Autodesk Inventor part; units mm, degrees
ref_plane "YZ Plane" through (0, 0, 0) normal (1, 0, 0) x (0, 1, 0)
ref_plane "XZ Plane" through (0, 0, 0) normal (0, 1, 0) x (-1, 0, 0)
ref_plane "XY Plane" through (0, 0, 0) normal (0, 0, 1) x (1, 0, 0)
sketch "Náčrt1" plane through (0, 0, 0) normal (0, 0, 1) x (1, 0, 0)
  line L0 (9.3423, 0) -> (16.6577, 0)
  line L1 (26, 28.3693) -> (26, 51.0917)
  line L2 (0, 51.0917) -> (0, 28.3693)
  circle A0 centre (13, 67) radius 10
  arc A1 (23.4879, 59.3186) -> (2.5121, 59.3186) centre (13, 67) ccw
  circle A2 centre (13, 8) radius 4.5
  line L3 (10, 43) -> (16, 43)
  line L4 (16, 43) -> (16, 33)
  line L5 (16, 33) -> (10, 33)
  line L6 (10, 33) -> (10, 43)
  line L7 (26, 51.0917) -> (26, 28.3693)
  line L8 (0, 28.3693) -> (0, 51.0917)
  line L9 (0.0896, 27.6417) -> (6.4319, 2.2724)
  line L10 (25.9104, 27.6417) -> (19.5681, 2.2724)
  line L11 (25.4962, 52.7558) -> (23.4121, 55.8819)
  line L12 (0.5038, 52.7558) -> (2.5879, 55.8819)
  arc A3 (6.4319, 2.2724) -> (9.3423, 0) centre (9.3423, 3) ccw
  arc A4 (16.6577, 0) -> (19.5681, 2.2724) centre (16.6577, 3) ccw
  arc A5 (0.5038, 52.7558) -> (0, 51.0917) centre (3, 51.0917) ccw
  arc A6 (26, 51.0917) -> (25.4962, 52.7558) centre (23, 51.0917) ccw
  arc A7 (23.4879, 59.3186) -> (23.4121, 55.8819) centre (25.9082, 57.546) ccw
  arc A8 (2.5879, 55.8819) -> (2.5121, 59.3186) centre (0.0918, 57.546) ccw
  arc A9 (25.9104, 27.6417) -> (26, 28.3693) centre (23, 28.3693) ccw
  arc A10 (0, 28.3693) -> (0.0896, 27.6417) centre (3, 28.3693) ccw
  point P0 (0, 0)
  point P1 (13, 38)
  point P2 (13, 38)
  point P3 (22.1538, 57.7692)
  point P4 (3.8462, 57.7692)
  dimension "d4" = 3
  dimension "d11" = 20
extrude "Vysunutí1" add sketch "Náčrt1" along normal blind 6
fillet "Zaoblení1" radius 1 16 edges at (25.8713, 51.961, 6) (24.4541, 54.3188, 6) (22.9089, 57.6122, 6) (13, 80, 6) (3.0911, 57.6122, 6) (1.5459, 54.3188, 6) (0.1287, 51.961, 6) (0, 39.7305, 6) (0.0225, 28.0028, 6) (3.2607, 14.9571, 6) (7.4961, 0.6354, 6) (13, 0, 6) (18.5039, 0.6354, 6) (22.7393, 14.9571, 6) (25.9775, 28.0028, 6) (26, 39.7305, 6)
fillet "Zaoblení2" radius 1 16 edges at (25.8713, 51.961, 0) (24.4541, 54.3188, 0) (22.9089, 57.6122, 0) (13, 80, 0) (3.0911, 57.6122, 0) (1.5459, 54.3188, 0) (0.1287, 51.961, 0) (0, 39.7305, 0) (0.0225, 28.0028, 0) (3.2607, 14.9571, 0) (7.4961, 0.6354, 0) (13, 0, 0) (18.5039, 0.6354, 0) (22.7393, 14.9571, 0) (25.9775, 28.0028, 0) (26, 39.7305, 0)
properties part number "crossguard"
Source: CAD feature listing. Evaluate the final solid. Frame: model axes, mm. A direction names the side the tool comes from. Give positions to 0.01 mm unless a question says otherwise; leave off trailing zeros. Write each loop counter-clockwise with the first axis right and the second up, starting at its lowest first coordinate (ties: lowest second). Pieces come first, ordered by that corner, then holes.
1. First-contact query: pin 1 (4 mm diameter, centred on x = 13.5, y = 8.5, fed in from -Z); pin 2 (5 mm diameter, centred on x = 5, y = 58.5, fed in from -Z); pin 3 (2 mm diameter, centred on x = 15.5, z = 4.5, fed in from +Y). Flat tips, straight axial feed; report the tip coordinate or a pass-through.
2. Section query D-D (y = 67). Return the cut outline in (x, z).
3. Access query for faces 4 (the face through (24.469, 54.297, 2.972)), 5 (the face through (13, 33, 3)), 6 (the face through (1.781, 54.13, 5.715)), 7 (the face through (0.125, 51.949, 2.972)), 8 (the face through (3.58, 14.85, 0.3)). Directions: +Z, -Z, +X, -X, +Y, -Y. A direction counts if a zero-diameter tool reaches every point of the face in a straight line with its end or side. Return the directions, or none.
4. Section query A-A (y = 39.5). Return the cut outline in (x, z), then the cut area to 3 significant figures.
5. Section query B-B (x = 13). Return the cut outline in (y, z).
6. Material intervals for line 1 along Y through (x, z) = (13, 2.5); line 2 along Y through (x, z) = (17.75, 0.75); line 3 along X through (y, z) = (26, 0.5), sorted ascending.
7. Section query C-C (z = 2.5). Return the cut outline in (x, y), then the cut area to 3 significant figures.
8. Pull-direction query (Y, two-part tool) for faces 1 (the face through (26, 40, 3)), 2 (the face through (3.09, 57.64, 2.97)), 3 (the face through (3.597, 14.852, 5.715)); classes: +Y half, -Y half, draft (parallel to the pull), parting line (faces both ways), or undercut.
Output values:
1. pin 1: passes through
1. pin 2: stops at z = 0
1. pin 3: stops at y = 79.91
2. outline: (0, 1) arc R1 ccw to (1, 0) - (3, 0) - (3, 6) - (1, 6) arc R1 ccw to (0, 5) - close; (23, 0) - (25, 0) arc R1 ccw to (26, 1) - (26, 5) arc R1 ccw to (25, 6) - (23, 6) - close
3. face 4: +Z, -Z, +X
3. face 5: +Z, -Z
3. face 6: +Z, -X
3. face 7: +Z, -Z, -X
3. face 8: -Z, -X, -Y
4. outline: (0, 1) arc R1 ccw to (1, 0) - (10, 0) - (10, 6) - (1, 6) arc R1 ccw to (0, 5) - close; (16, 0) - (25, 0) arc R1 ccw to (26, 1) - (26, 5) arc R1 ccw to (25, 6) - (16, 6) - close
4. area: 119 mm2
5. outline: (0, 1) arc R1 ccw to (1, 0) - (3.5, 0) - (3.5, 6) - (1, 6) arc R1 ccw to (0, 5) - close; (12.5, 0) - (33, 0) - (33, 6) - (12.5, 6) - close; (43, 0) - (57, 0) - (57, 6) - (43, 6) - close; (77, 0) - (79, 0) arc R1 ccw to (80, 1) - (80, 5) arc R1 ccw to (79, 6) - (77, 6) - close
6. line 1: y = 0 to 3.5, 12.5 to 33, 43 to 57, 77 to 80
6. line 2: y = 0.24 to 58.2, 75.8 to 79.07
6. line 3: x = 0.64 to 25.36
7. outline: (0, 28.37) arc R3 ccw to (0.09, 27.64) - (6.43, 2.27) arc R3 ccw to (9.34, 0) - (16.66, 0) arc R3 ccw to (19.57, 2.27) - (25.91, 27.64) arc R3 ccw to (26, 28.37) - (26, 51.09) arc R3 ccw to (25.5, 52.76) - (23.41, 55.88) arc R3 cw to (23.49, 59.32) arc R13 ccw (long way) to (2.51, 59.32) arc R3 cw to (2.59, 55.88) - (0.5, 52.76) arc R3 ccw to (0, 51.09) - close; hole circle Ø20 at (13, 67); hole circle Ø9 at (13, 8); hole (10, 33) - (16, 33) - (16, 43) - (10, 43) - close
7. area: 1,330 mm2
8. face 1: draft
8. face 2: undercut
8. face 3: -Y half
